Geometry check sheet. Reference: the model listing, model coordinates, mm. Face numbers are marked on the shaded views. A direction names the side the tool comes from. Round coordinates to 2 decimals unless told otherwise and drop trailing zeros. Order: outer loops, then holes, each group sorted by start corner. A loop starts at its lowest first (then second) coordinate and runs counter-clockwise, first axis right, second up. Notation, with made-up numbers: (15, 46.25) - (61, 46.25) arc R19 ccw to (61, 65.25) - close; hole circle Ø7 at (89.25, 87.5). An arc over 180 degrees is marked (long way). Return JSON: item names as keys, results as strings. Group by question number.
Q1. Sectioned sample at C-C, the plane x = 14. Record the cut outline in (y, z).
Q2. Draft check along X on the marked faces 1 and 2. Enter one of: pulls with the +X half, pulls with the -X half, needs draft (parallel to the pull), parting line crosses it, or undercut.
Q3. Material ranges on line 1 along X through (y, z) = (21, 6); line 2 along Z through (x, y) = (22, -14.5); line 3 along Z through (x, y) = (-7.5, 21), recorded low to high.
Q4. Gauge pin test, flat ends, axial feed: pin 1 Ø13.5 at (x, y) = (-7.5, -17) entering from +Z; pin 2 Ø10 at (x, y) = (-12, 3) entering from +Z. Record the tip position at first contact, or that the pin passes through.
Q5. Sectioned sample at A-A, the plane y = 5. Record the cut outline in (x, z), then the cut area to 3 significant figures.
Q6. Sectioned sample at B-B, the plane z = 4.75. Record the cut outline in (x, y), then the cut area to 3 significant figures.
Q7. Tool access check on the marked faces 3 and 4. Record the directions out of +Z, -Z, +X, -X, +Y, -Y that give a thin tool (end or side, any length) a straight path to the whole face; none if there is none.
Q8. Sectioned sample at D-D, the plane y = -18.5. Record the cut outline in (x, z).
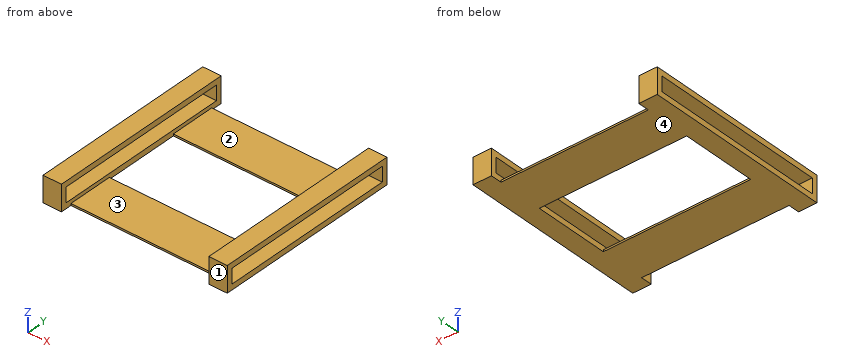
```python
from build123d import *

# Parameters (mm, degrees)
F1_START      = 20
F0_W          = 48
F0_H          = 4
F0_W_2        = 12.2445234573
F0_H_2        = 0.5
F1_DEPTH      = 5
F2_START      = -20
F2_DEPTH      = 5
F3_DEPTH      = 25
F3_DEPTH_BACK = 25


with BuildPart() as f1:
    # F0 (on Right) → F1 (new body)
    with BuildSketch(Plane.YZ.offset(F1_START)):
        Polygon((-25.5, 7), (-25.5, 0), (-22.4627573043, 0), (-22.4627573043, 0.5), (-10.218233847, 0.5), (-10.218233847, 0), (10.218233847, 0), (10.218233847, 0.5), (22.4627573043, 0.5), (22.4627573043, 0), (25.5, 0), (25.5, 7), align=None)
        with Locations((0, 3.5)):
            Rectangle(F0_W, F0_H, mode=Mode.SUBTRACT)
        with Locations((-16.3404955757, 0.25)):
            Rectangle(F0_W_2, F0_H_2)
        with Locations((16.3404955757, 0.25)):
            Rectangle(F0_W_2, F0_H_2)
    extrude(amount=F1_DEPTH)



with BuildPart() as f2:
    # F0 (on Right) → F2 (new body)
    with BuildSketch(Plane.YZ.offset(F2_START)):
        Polygon((-25.5, 7), (-25.5, 0), (-22.4627573043, 0), (-22.4627573043, 0.5), (-10.218233847, 0.5), (-10.218233847, 0), (10.218233847, 0), (10.218233847, 0.5), (22.4627573043, 0.5), (22.4627573043, 0), (25.5, 0), (25.5, 7), align=None)
        with Locations((0, 3.5)):
            Rectangle(F0_W, F0_H, mode=Mode.SUBTRACT)
        with Locations((-16.3404955757, 0.25)):
            Rectangle(F0_W_2, F0_H_2)
        with Locations((16.3404955757, 0.25)):
            Rectangle(F0_W_2, F0_H_2)
    extrude(amount=-F2_DEPTH)


with BuildPart() as f1_1:
    add(f1.part)

    add(f2.part)  # F3 merges F2
    # F0 (on Right) → F3 (join, two sides)
    with BuildSketch(Plane.YZ) as f3_sk:
        with Locations((16.3404955757, 0.25)):
            Rectangle(F0_W_2, F0_H_2)
        with Locations((-16.3404955757, 0.25)):
            Rectangle(F0_W_2, F0_H_2)
    extrude(amount=F3_DEPTH)
    extrude(f3_sk.sketch, amount=-F3_DEPTH_BACK)


solid = f1_1.part
```
Reply:
{
 "1": {"outline": "(-22.46, 0) - (-10.22, 0) - (-10.22, 0.5) - (-22.46, 0.5) - close; (10.22, 0) - (22.46, 0) - (22.46, 0.5) - (10.22, 0.5) - close"},
 "2": {"face 1": "needs draft", "face 2": "undercut"},
 "3": {"line 1": "-25 to -20, 20 to 25", "line 2": "0 to 1.5, 5.5 to 7", "line 3": "0 to 0.5"},
 "4": {"pin 1": "z = 0.5", "pin 2": "through"},
 "5": {"outline": "(-25, 0) - (-20, 0) - (-20, 1.5) - (-25, 1.5) - close; (-25, 5.5) - (-20, 5.5) - (-20, 7) - (-25, 7) - close; (20, 0) - (25, 0) - (25, 1.5) - (20, 1.5) - close; (20, 5.5) - (25, 5.5) - (25, 7) - (20, 7) - close", "area": "30.0 mm^2"},
 "6": {"outline": "(-25, -25.5) - (-20, -25.5) - (-20, -24) - (-25, -24) - close; (-25, 24) - (-20, 24) - (-20, 25.5) - (-25, 25.5) - close; (20, -25.5) - (25, -25.5) - (25, -24) - (20, -24) - close; (20, 24) - (25, 24) - (25, 25.5) - (20, 25.5) - close", "area": "30.0 mm^2"},
 "7": {"face 3": "+Z, +Y, -Y", "face 4": "-Z, +X, -X, +Y, -Y"},
 "8": {"outline": "(-25, 0) - (25, 0) - (25, 1.5) - (20, 1.5) - (20, 0.5) - (-20, 0.5) - (-20, 1.5) - (-25, 1.5) - close; (-25, 5.5) - (-20, 5.5) - (-20, 7) - (-25, 7) - close; (20, 5.5) - (25, 5.5) - (25, 7) - (20, 7) - close"}
}
